from build123d import *

# Parameters (mm, degrees)
SKETCH1_W           = 55
SKETCH1_H           = 112
BOSS_EXTRUDE1_DEPTH = 160
CUT_EXTRUDE1_REACH  = 204.901
SKETCH2_W           = 148
SKETCH2_H           = 102
CUT_EXTRUDE2_REACH  = 198.655
SKETCH3_R           = 9
SKETCH3_R_2         = 3.05
CUT_EXTRUDE4_DEPTH  = 4
CUT_EXTRUDE11_REACH = 204.901
SKETCH15_R          = 2.075
CUT_EXTRUDE12_DEPTH = 3.2
CUT_EXTRUDE14_REACH = 204.901
SKETCH17_W          = 18
SKETCH17_H          = 9.5
CUT_EXTRUDE15_REACH = 204.901
SKETCH19_R          = 2.075
CUT_EXTRUDE16_DEPTH = 2


with BuildPart() as part:
    # Sketch1 → Boss-Extrude1 (new body)
    with BuildSketch(Plane(origin=(0, 0, 0), x_dir=(0, 0, -1), z_dir=(1, 0, 0))):
        with Locations((27.5, -56)):
            Rectangle(SKETCH1_W, SKETCH1_H)
    extrude(amount=BOSS_EXTRUDE1_DEPTH)

    # Sketch2 → Cut-Extrude1 (cut, up to next)
    with BuildSketch(Plane.XY, mode=Mode.PRIVATE) as cut_extrude1_sk1:
        with Locations((78, -55)):
            Rectangle(SKETCH2_W, SKETCH2_H)
    cut_extrude1_tool1 = extrude(cut_extrude1_sk1.sketch, amount=-CUT_EXTRUDE1_REACH, mode=Mode.PRIVATE) & part.part
    add(cut_extrude1_tool1.solids().sort_by_distance((78, -55, 0))[0], mode=Mode.SUBTRACT)

    # Sketch3 → Cut-Extrude2 (cut, up to next)
    with BuildSketch(Plane.ZY.offset(-152), mode=Mode.PRIVATE) as cut_extrude2_sk1:
        with Locations((-27.5, -39)):
            Circle(SKETCH3_R)
    cut_extrude2_tool1 = extrude(cut_extrude2_sk1.sketch, amount=-CUT_EXTRUDE2_REACH, mode=Mode.PRIVATE) & part.part
    # Sketch3 → Cut-Extrude2 (cut, up to next)
    with BuildSketch(Plane.ZY.offset(-152), mode=Mode.PRIVATE) as cut_extrude2_sk2:
        with Locations((-27.5, -15)):
            Circle(SKETCH3_R_2)
    cut_extrude2_tool2 = extrude(cut_extrude2_sk2.sketch, amount=-CUT_EXTRUDE2_REACH, mode=Mode.PRIVATE) & part.part
    # Sketch3 → Cut-Extrude2 (cut, up to next)
    with BuildSketch(Plane.ZY.offset(-152), mode=Mode.PRIVATE) as cut_extrude2_sk3:
        with Locations(Location((-27.5, -63, 0), (0, 0, 180))):
            Circle(SKETCH3_R_2)
    cut_extrude2_tool3 = extrude(cut_extrude2_sk3.sketch, amount=-CUT_EXTRUDE2_REACH, mode=Mode.PRIVATE) & part.part
    add(cut_extrude2_tool1.solids().sort_by_distance((152, -39, -27.5))[0], mode=Mode.SUBTRACT)
    add(cut_extrude2_tool2.solids().sort_by_distance((152, -15, -27.5))[0], mode=Mode.SUBTRACT)
    add(cut_extrude2_tool3.solids().sort_by_distance((152, -63, -27.5))[0], mode=Mode.SUBTRACT)

    # Sketch6 → Cut-Extrude4 (cut)
    with BuildSketch(Plane(origin=(160, 0, 0), x_dir=(0, 0, -1), z_dir=(1, 0, 0))):
        Polygon((30.386751346, -20), (33.273502692, -15), (30.386751346, -10), (24.613248654, -10), (21.726497308, -15), (24.613248654, -20), align=None)
        Polygon((30.386751346, -68), (33.273502692, -63), (30.386751346, -58), (24.613248654, -58), (21.726497308, -63), (24.613248654, -68), align=None)
    extrude(amount=-CUT_EXTRUDE4_DEPTH, mode=Mode.SUBTRACT)

    # Sketch15 → Cut-Extrude11 (cut, up to next)
    with BuildSketch(Plane(origin=(0, -112, 0), x_dir=(-1, 0, 0), z_dir=(0, -1, 0)), mode=Mode.PRIVATE) as cut_extrude11_sk1:
        with Locations(Location((-34.5, 9, 0), (0, 0, 90))):
            Circle(SKETCH15_R)
    cut_extrude11_tool1 = extrude(cut_extrude11_sk1.sketch, amount=-CUT_EXTRUDE11_REACH, mode=Mode.PRIVATE) & part.part
    # Sketch15 → Cut-Extrude11 (cut, up to next)
    with BuildSketch(Plane(origin=(0, -112, 0), x_dir=(-1, 0, 0), z_dir=(0, -1, 0)), mode=Mode.PRIVATE) as cut_extrude11_sk2:
        with Locations(Location((-74.5, 9, 0), (0, 0, 90))):
            Circle(SKETCH15_R)
    cut_extrude11_tool2 = extrude(cut_extrude11_sk2.sketch, amount=-CUT_EXTRUDE11_REACH, mode=Mode.PRIVATE) & part.part
    # Sketch15 → Cut-Extrude11 (cut, up to next)
    with BuildSketch(Plane(origin=(0, -112, 0), x_dir=(-1, 0, 0), z_dir=(0, -1, 0)), mode=Mode.PRIVATE) as cut_extrude11_sk3:
        with Locations(Location((-74.5, 46, 0), (0, 0, 90))):
            Circle(SKETCH15_R)
    cut_extrude11_tool3 = extrude(cut_extrude11_sk3.sketch, amount=-CUT_EXTRUDE11_REACH, mode=Mode.PRIVATE) & part.part
    # Sketch15 → Cut-Extrude11 (cut, up to next)
    with BuildSketch(Plane(origin=(0, -112, 0), x_dir=(-1, 0, 0), z_dir=(0, -1, 0)), mode=Mode.PRIVATE) as cut_extrude11_sk4:
        with Locations(Location((-34.5, 46, 0), (0, 0, 90))):
            Circle(SKETCH15_R)
    cut_extrude11_tool4 = extrude(cut_extrude11_sk4.sketch, amount=-CUT_EXTRUDE11_REACH, mode=Mode.PRIVATE) & part.part
    add(cut_extrude11_tool1.solids().sort_by_distance((34.5, -112, -9))[0], mode=Mode.SUBTRACT)
    add(cut_extrude11_tool2.solids().sort_by_distance((74.5, -112, -9))[0], mode=Mode.SUBTRACT)
    add(cut_extrude11_tool3.solids().sort_by_distance((74.5, -112, -46))[0], mode=Mode.SUBTRACT)
    add(cut_extrude11_tool4.solids().sort_by_distance((34.5, -112, -46))[0], mode=Mode.SUBTRACT)

    # Sketch16 → Cut-Extrude12 (cut)
    with BuildSketch(Plane(origin=(0, -112, 0), x_dir=(-1, 0, 0), z_dir=(0, -1, 0))):
        Polygon((-38.541451884, 9), (-36.520725942, 5.5), (-32.479274058, 5.5), (-30.458548116, 9), (-32.479274058, 12.5), (-36.520725942, 12.5), align=None)
        Polygon((-76.520725942, 12.5), (-78.541451884, 9), (-76.520725942, 5.5), (-72.479274058, 5.5), (-70.458548116, 9), (-72.479274058, 12.5), align=None)
        Polygon((-72.479274058, 42.5), (-76.520725942, 42.5), (-78.541451884, 46), (-76.520725942, 49.5), (-72.479274058, 49.5), (-70.458548116, 46), align=None)
        Polygon((-36.520725942, 42.5), (-38.541451884, 46), (-36.520725942, 49.5), (-32.479274058, 49.5), (-30.458548116, 46), (-32.479274058, 42.5), align=None)
    extrude(amount=-CUT_EXTRUDE12_DEPTH, mode=Mode.SUBTRACT)

    # Sketch17 → Cut-Extrude14 (cut, up to next)
    with BuildSketch(Plane(origin=(0, 0, 0), x_dir=(1, 0, 0), z_dir=(0, 1, 0)), mode=Mode.PRIVATE) as cut_extrude14_sk1:
        with Locations((63, 50.25)):
            Rectangle(SKETCH17_W, SKETCH17_H)
    cut_extrude14_tool1 = extrude(cut_extrude14_sk1.sketch, amount=-CUT_EXTRUDE14_REACH, mode=Mode.PRIVATE) & part.part
    # Sketch17 → Cut-Extrude14 (cut, up to next)
    with BuildSketch(Plane(origin=(0, 0, 0), x_dir=(1, 0, 0), z_dir=(0, 1, 0)), mode=Mode.PRIVATE) as cut_extrude14_sk2:
        with Locations((63, 4.75)):
            Rectangle(SKETCH17_W, SKETCH17_H)
    cut_extrude14_tool2 = extrude(cut_extrude14_sk2.sketch, amount=-CUT_EXTRUDE14_REACH, mode=Mode.PRIVATE) & part.part
    add(cut_extrude14_tool1.solids().sort_by_distance((63, 0, -50.25))[0], mode=Mode.SUBTRACT)
    add(cut_extrude14_tool2.solids().sort_by_distance((63, 0, -4.75))[0], mode=Mode.SUBTRACT)

    # Sketch19 → Cut-Extrude15 (cut, up to next)
    with BuildSketch(Plane(origin=(0, 0, 0), x_dir=(1, 0, 0), z_dir=(0, 1, 0)), mode=Mode.PRIVATE) as cut_extrude15_sk1:
        with Locations(Location((63, 38.5, 0), (0, 0, 270))):
            Circle(SKETCH19_R)
    cut_extrude15_tool1 = extrude(cut_extrude15_sk1.sketch, amount=-CUT_EXTRUDE15_REACH, mode=Mode.PRIVATE) & part.part
    # Sketch19 → Cut-Extrude15 (cut, up to next)
    with BuildSketch(Plane(origin=(0, 0, 0), x_dir=(1, 0, 0), z_dir=(0, 1, 0)), mode=Mode.PRIVATE) as cut_extrude15_sk2:
        with Locations(Location((63, 16.5, 0), (0, 0, 270))):
            Circle(SKETCH19_R)
    cut_extrude15_tool2 = extrude(cut_extrude15_sk2.sketch, amount=-CUT_EXTRUDE15_REACH, mode=Mode.PRIVATE) & part.part
    add(cut_extrude15_tool1.solids().sort_by_distance((63, 0, -38.5))[0], mode=Mode.SUBTRACT)
    add(cut_extrude15_tool2.solids().sort_by_distance((63, 0, -16.5))[0], mode=Mode.SUBTRACT)

    # Sketch20 → Cut-Extrude16 (cut)
    with BuildSketch(Plane.XZ.offset(4)):
        Polygon((67.041451884, -16.5), (65.020725942, -13), (60.979274058, -13), (58.958548116, -16.5), (60.979274058, -20), (65.020725942, -20), align=None)
        Polygon((65.020725942, -35), (67.041451884, -38.5), (65.020725942, -42), (60.979274058, -42), (58.958548116, -38.5), (60.979274058, -35), align=None)
    extrude(amount=-CUT_EXTRUDE16_DEPTH, mode=Mode.SUBTRACT)


solid = part.part
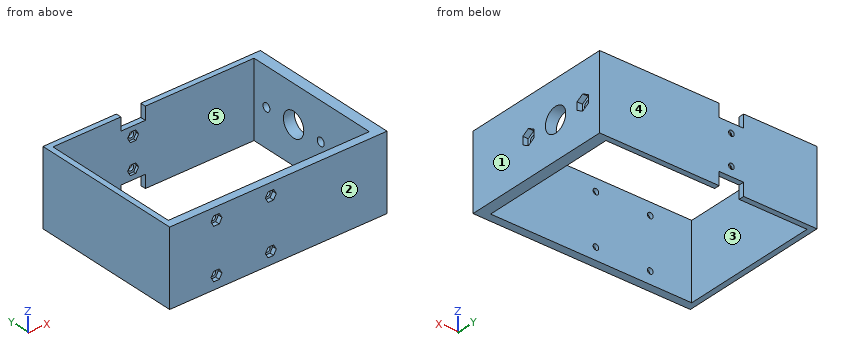
The listing builds one solid part. Answer for the finished solid, in the listing's coordinates (mm). Face numbers are marked on the shaded views. A direction names the side the tool comes from. Give positions to 0.01 mm unless a question says otherwise; leave off trailing zeros. Order: outer loops, then holes, each group sorted by start corner. A loop starts at its lowest first (then second) coordinate and runs counter-clockwise, first axis right, second up. Notation, with made-up numbers: (30, 78.25) -> (77, 78.25) arc R24 cw to (77, 90.25) -> close; hole circle Ø3 at (73.5, 28). An arc over 180 degrees is marked (long way). Put each result on its own line as item: value.
Item 1: A cutting plane is placed at A-A on x = 74.5. Give the vertices of the cut face in (y, z) (3 decimals), plus the area to 3 significant figures.
Established:
outline: (-112, -55) -> (-106, -55) -> (-106, -48.075) -> (-108.8, -48.075) -> (-108.8, -49.5) -> (-112, -49.5) -> close; (-112, -42.5) -> (-108.8, -42.5) -> (-108.8, -43.925) -> (-106, -43.925) -> (-106, -11.075) -> (-108.8, -11.075) -> (-108.8, -12.5) -> (-112, -12.5) -> close; (-112, -5.5) -> (-108.8, -5.5) -> (-108.8, -6.925) -> (-106, -6.925) -> (-106, 0) -> (-112, 0) -> close; (-4, -55) -> (0, -55) -> (0, 0) -> (-4, 0) -> close
area: 482 mm^2
Item 2: A cutting plane is placed at D-D on x = 141.5. Give the vertices of the cut face in (y, z).
Established:
outline: (-112, -55) -> (-106, -55) -> (-106, 0) -> (-112, 0) -> close; (-4, -55) -> (0, -55) -> (0, 0) -> (-4, 0) -> close
Item 3: A cutting plane is placed at C-C on y = -39. Give the vertices of the cut face in (x, z), plus the area to 3 significant figures.
Established:
outline: (0, -55) -> (4, -55) -> (4, 0) -> (0, 0) -> close; (152, -55) -> (160, -55) -> (160, -36.5) -> (152, -36.5) -> close; (152, -18.5) -> (160, -18.5) -> (160, 0) -> (152, 0) -> close
area: 516 mm^2
Item 4: Straight lines are drawn through the part: line 1 (X direction, y = -71, z = -11); line 2 (X direction, y = -0.95, z = -16.5) (3 decimals); line 3 (Y direction, x = 26, z = -41.5). For each, find the intervals that lie inside material, in ascending order.
Established:
line 1: x = 0 to 4, 152 to 160
line 2: x = 0 to 60.925, 65.075 to 160
line 3: y = -112 to -106, -4 to 0
Item 5: For a pull along X with two mould halves and no side action, classify the marked faces 1, 2 and 3 as released by +X, released by -X, zero draft, split by the parting line, or undercut.
Established:
face 1: released by +X
face 2: zero draft
face 3: undercut
Item 6: A cutting plane is placed at B-B on z = -27.5. Give the vertices of the cut face in (x, y), plus the area to 3 significant figures.
Established:
outline: (0, -112) -> (160, -112) -> (160, -68) -> (156, -68) -> (156, -66.05) -> (152, -66.05) -> (152, -106) -> (4, -106) -> (4, -4) -> (152, -4) -> (152, -11.95) -> (156, -11.95) -> (156, -10) -> (160, -10) -> (160, 0) -> (0, 0) -> close; (152, -59.95) -> (156, -59.95) -> (156, -58) -> (160, -58) -> (160, -48) -> (152, -48) -> close; (152, -30) -> (160, -30) -> (160, -20) -> (156, -20) -> (156, -18.05) -> (152, -18.05) -> close
area: 2,550 mm^2
Item 7: Given P1, Ø16, axis at y = -39, z = -27.5, coming from the +X side; P2, Ø2, axis at x = 74, z = -10, coming from the -Y side; P3, Ø8, axis at y = -63, z = -27.5, coming from the +X side, each flat-ended and moving along its own axis, determine where each tip first touches the part or whether it passes through.
Established:
P1: stops at x = 4
P2: stops at y = -108.8
P3: stops at x = 156
Item 8: For the marked faces 4 and 5, determine the directions among +Z, -Z, +X, -X, +Y, -Y from which every point of the face is accessible in a straight line to the end or side of a thin tool.
Established:
face 4: +Z, -Z, +X, -X, +Y
face 5: +Z, -Z
